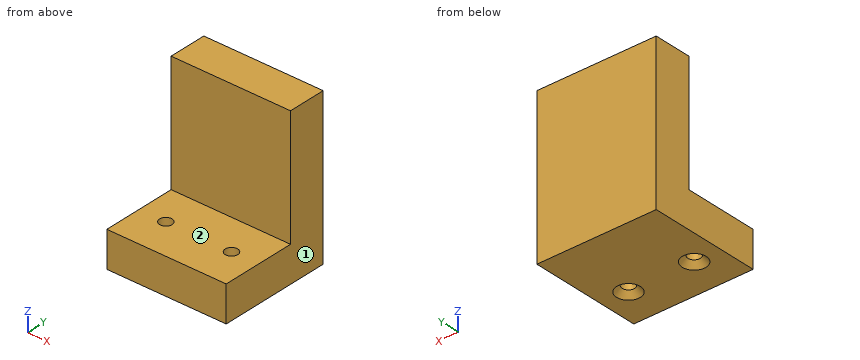
```python
from build123d import *

# Parameters (mm, degrees)
F0_W           = 40
F0_H           = 52
F1_DEPTH       = 37.7
F2_W           = 40
F2_H           = 40
F3_DEPTH       = 25
F5_D           = 4.2
F5_CSINK_D     = 8
F5_CSINK_ANGLE = 90


with BuildPart() as f1:
    # F0 (on Front) → F1 (new body)
    with BuildSketch(Plane.XZ):
        with Locations((20, 26)):
            Rectangle(F0_W, F0_H)
    extrude(amount=F1_DEPTH)

    # F2 (on face) → F3 (cut)
    with BuildSketch(Plane.XZ.offset(37.7)):
        with Locations((20, 32)):
            Rectangle(F2_W, F2_H)
    extrude(amount=-F3_DEPTH, mode=Mode.SUBTRACT)

    # F5 (through all)
    with Locations(Plane(origin=(0, 0, 0), x_dir=(1, 0, 0), z_dir=(0, 0, -1))):
        with Locations((9, 25.2), (31, 25.2)):
            CounterSinkHole(F5_D / 2, F5_CSINK_D / 2, counter_sink_angle=F5_CSINK_ANGLE)


solid = f1.part
```
Work out the finished part from the listing and answer in its coordinate system (mm). Face numbers are marked on the shaded views. A direction names the side the tool comes from. Give positions to 0.01 mm unless a question says otherwise; leave off trailing zeros. Order: outer loops, then holes, each group sorted by start corner. A loop starts at its lowest first (then second) coordinate and runs counter-clockwise, first axis right, second up. Notation, with made-up numbers: (17, -21.5) -> (49, -21.5) arc R30 ccw to (49, 2.5) -> close; hole circle Ø6 at (-8, 49.25). An arc over 180 degrees is marked (long way). Answer as CSV lines item,"result". Start each with the question number.
(1) Section C-C, the plane z = 36.5 is taken. Write down the section's boundary in (x, y), plus the area to 3 significant figures.
(2) Which of the six approach directions +Z, -Z, +X, -X, +Y, -Y give full straight-line access (tool end or side, diameter ignored) to the marked faces 1 and 2?
(3) Section B-B, the plane x = 9 is taken. Write down the section's boundary in (y, z), plus the area to 3 significant figures.
(4) Section A-A, the plane y = -25.2 is taken. Write down the section's boundary in (x, z), plus the area to 3 significant figures.
(5) Consider line 1 along X through (y, z) = (-25, 9); line 2 along Y through (x, z) = (31, 5); line 3 along Y through (x, z) = (4, 38.5). Determine where each line is inside the solid, lowest interval first.
(6) Section D-D, the plane x = 23 is taken. Write down the section's boundary in (y, z).
(7) Each of these flat-tipped pins is pushed along its axis until it touches: pin 1 Ø10 at (x, z) = (15, 46.5) entering from +Y; pin 2 Ø12.5 at (x, y) = (16.5, -24.5) entering from +Z. Where does it stop, or does it pass through?
Entries:
1,outline,"(0, -12.7) -> (40, -12.7) -> (40, 0) -> (0, 0) -> close"
1,area,"508 mm²"
2,face 1,"+Z, -Z, +X, +Y, -Y"
2,face 2,"+Z, +X, -X, -Y"
3,outline,"(-37.7, 0) -> (-29.2, 0) -> (-27.3, 1.9) -> (-27.3, 12) -> (-37.7, 12) -> close; (-23.1, 1.9) -> (-21.2, 0) -> (0, 0) -> (0, 52) -> (-12.7, 52) -> (-12.7, 12) -> (-23.1, 12) -> close"
3,area,"906 mm²"
4,outline,"(0, 0) -> (5, 0) -> (6.9, 1.9) -> (6.9, 12) -> (0, 12) -> close; (11.1, 1.9) -> (13, 0) -> (27, 0) -> (28.9, 1.9) -> (28.9, 12) -> (11.1, 12) -> close; (33.1, 1.9) -> (35, 0) -> (40, 0) -> (40, 12) -> (33.1, 12) -> close"
4,area,"372 mm²"
5,line 1,"0 to 6.91, 11.09 to 28.91, 33.09 to 40"
5,line 2,"-37.7 to -27.3, -23.1 to 0"
5,line 3,"-12.7 to 0"
6,outline,"(-37.7, 0) -> (0, 0) -> (0, 52) -> (-12.7, 52) -> (-12.7, 12) -> (-37.7, 12) -> close"
7,pin 1,"y = 0"
7,pin 2,"z = 12"
